from build123d import *

# Parameters (mm, degrees)
BOSS_EXTRUDE1_START                       = 12.7
BOSS_EXTRUDE1_DEPTH                       = 12.7
BOSS_EXTRUDE2_DEPTH                       = 12.7
SKETCH7_R                                 = 0.9525
CUT_EXTRUDE1_DEPTH                        = 111.090903984
SKETCH10_R                                = 0.9525
CUT_EXTRUDE2_DEPTH                        = 110.494104933
CSK_FOR_6_FLAT_HEAD_MACHINE_SCREW_2_COUNT = 2
CSK_FOR_6_FLAT_HEAD_MACHINE_SCREW_2_PITCH = 11.43


with BuildPart() as part:
    # Sweep1: sweep along a path in Sketch4
    with BuildLine(Plane.XY) as sweep1_path:
        Line((0, 0), (0, -92.964))
    # Sketch3 → Sweep1 (sweep)
    with BuildSketch(Plane(origin=(0, 0, 0), x_dir=(1, 0, 0), z_dir=(0, 1, 0))):
        with BuildLine():
            Line((0, 16.62500014), (-25.4, 16.62500014))
            Line((-25.4, 16.62500014), (-25.4, 10.27500014))
            Line((-25.4, 10.27500014), (-6.985, 10.27500014))
            ThreePointArc((-6.985, 10.27500014), (-6.535987194, 10.089012946), (-6.35, 9.64000014))
            Line((-6.35, 9.64000014), (-6.35, -14.48999986))
            ThreePointArc((-6.35, -14.48999986), (-6.535987194, -14.939012666), (-6.985, -15.12499986))
            Line((-6.985, -15.12499986), (-25.4, -15.12499986))
            Line((-25.4, -15.12499986), (-25.4, -21.47499986))
            Line((-25.4, -21.47499986), (0, -21.47499986))
            Line((0, -21.47499986), (0, 16.62500014))
        make_face()
    sweep(path=sweep1_path.line)

    # Sketch5 → Boss-Extrude1 (add)
    with BuildSketch(Plane.XZ.offset(92.964).offset(BOSS_EXTRUDE1_START)):
        with BuildLine():
            Line((-25.4, 18.04599986), (-3.429, 18.04599986))
            Line((-3.429, 18.04599986), (-3.429, -13.19600014))
            Line((-3.429, -13.19600014), (-25.4, -13.19600014))
            Line((-25.4, -13.19600014), (-25.4, -10.27500014))
            Line((-25.4, -10.27500014), (-6.985, -10.27500014))
            ThreePointArc((-6.985, -10.27500014), (-6.535987194, -10.089012946), (-6.35, -9.64000014))
            Line((-6.35, -9.64000014), (-6.35, 14.48999986))
            ThreePointArc((-6.35, 14.48999986), (-6.535987194, 14.939012666), (-6.985, 15.12499986))
            Line((-6.985, 15.12499986), (-25.4, 15.12499986))
            Line((-25.4, 15.12499986), (-25.4, 18.04599986))
        make_face()
    extrude(amount=-BOSS_EXTRUDE1_DEPTH)

    # Sketch6 → Boss-Extrude2 (add)
    with BuildSketch(Plane(origin=(0, 0, 0), x_dir=(1, 0, 0), z_dir=(0, 1, 0))):
        Polygon((-25.4, 13.45000014), (-25.4, 16.62500014), (0, 16.62500014), (0, -21.47499986), (-25.4, -21.47499986), (-25.4, -18.29999986), (-3.175, -18.29999986), (-3.175, 13.45000014), align=None)
    extrude(amount=BOSS_EXTRUDE2_DEPTH)

    # Sketch7 → Cut-Extrude1 (cut, through all)
    with BuildSketch(Plane.ZY.offset(3.175)):
        with Locations((-3.29000014, 6.35)):
            Circle(SKETCH7_R)
        with Locations((8.13999986, 6.35)):
            Circle(SKETCH7_R)
    extrude(amount=-CUT_EXTRUDE1_DEPTH, mode=Mode.SUBTRACT)

    # Sketch10 → Cut-Extrude2 (cut, through all)
    with BuildSketch(Plane.ZY.offset(6.35)):
        with Locations((-3.29000014, -99.314)):
            Circle(SKETCH10_R)
        with Locations((8.13999986, -99.314)):
            Circle(SKETCH10_R)
    extrude(amount=-CUT_EXTRUDE2_DEPTH, mode=Mode.SUBTRACT)

    # Sketch13 → CSK for #6 Flat Head Machine Screw (100)2 (revolve, cut)
    with BuildSketch(Plane(origin=(-6.35, -99.314, -3.29000014), x_dir=(0, 0, 1), z_dir=(0, 1, 0))):
        Polygon((0, 0), (0, 2.563442612), (2.15265, 1.27), (2.15265, 1.166893902), (3.5433, 0), align=None)
    csk_for_6_flat_head_machine_screw_100 = revolve(axis=Axis((-12.7, -99.314, -3.29000014), (1, 0, 0)), mode=Mode.SUBTRACT)

    # CSK for _6 Flat Head Machine Screw _ 2: CSK for #6 Flat Head Machine Screw (100)2 ×2
    with Locations(*[(0, 0, i * CSK_FOR_6_FLAT_HEAD_MACHINE_SCREW_2_PITCH) for i in range(1, CSK_FOR_6_FLAT_HEAD_MACHINE_SCREW_2_COUNT)]):
        add(csk_for_6_flat_head_machine_screw_100, mode=Mode.SUBTRACT)


solid = part.part
Model file for the job. Use its own axes, mm. A direction names the side the tool comes from. Coordinates: 2 decimals unless noted, no trailing zeros. Order: outer loops, then holes, each group sorted by start corner. A loop starts at its lowest first (then second) coordinate and runs counter-clockwise, first axis right, second up. Notation, with made-up numbers: M 64.5,3.25 L 79.5,3.25 A32 ccw 79.5,29.25 Z; hole C 43,2 d11. An arc over 180 degrees is marked long. Return JSON: item names as keys, results as strings.
1. Tool access for faces 1 (the face through (-3.175, 6, 3)), 2 (the face through (-3.429, -99, 3)), 3 (the face through (-6.35, -54, 2)): list every direction of +Z, -Z, +X, -X, +Y, -Y with a clear straight run to the whole face (end or side of a thin tool).
Ans:
{"face 1": "-X, +Y", "face 2": "+Z, -Z, +X, -Y", "face 3": "-X, +Y, -Y"}
2. Saw through at A-A (x = -9.25). Give the cut face in (y, z) (3 decimals).
Ans:
{"outline": "M -105.664,-13.196 L -92.964,-13.196 L -92.964,-16.625 L 12.7,-16.625 L 12.7,-13.45 L 0,-13.45 L 0,-10.275 L -105.664,-10.275 Z; M -105.664,15.125 L 0,15.125 L 0,18.3 L 12.7,18.3 L 12.7,21.475 L -92.964,21.475 L -92.964,18.046 L -105.664,18.046 Z"}
3. Pull direction Z, two halves, no side cores. Call faces 4 (the face through (-25.4, -47, 18)), 5 (the face through (-1.61, 5.99, 9.02)), 6 (the face through (-15, -99, 18.046)), 7 (the face through (-14, 6, 18.3)): +Z half, -Z half, draft (parallel to the pull), parting line (faces both ways), or undercut.
Ans:
{"face 4": "draft", "face 5": "undercut", "face 6": "+Z half", "face 7": "undercut"}
4. Flat gauge pins, fed straight in: pin 1 (3 mm diameter, centred on y = 6.35, z = -3.29, fed in from -X) (3 decimals); pin 2 (5 mm diameter, centred on y = -99.314, z = -3.29, fed in from +X); pin 3 (10 mm diameter, centred on x = -22.5, z = -8, fed in from +Y). Where does each tip first touch, or does it go through?
Ans:
{"pin 1": "x = -3.175", "pin 2": "x = -3.43", "pin 3": "y = 0"}
5. Drill centre lines: probe 1 along Y at (x, z) = (-0.85, -3.29); probe 2 along Z at (x, y) = (-19.25, -17) (3 decimals); probe 3 along Y at (x, z) = (-5.15, -3.29). Where is each one in solid material? Low to high.
Ans:
{"probe 1": "-92.96 to 5.4, 7.3 to 12.7", "probe 2": "-16.625 to -10.275, 15.125 to 21.475", "probe 3": "-105.66 to -101.47, -97.16 to 0"}
6. Saw through at B-B (z = 13). Give the cut face in (x, y) (3 decimals), and give its area (3 significant figures).
Ans:
{"outline": "M -6.35,-105.664 L -3.429,-105.664 L -3.429,-92.964 L 0,-92.964 L 0,12.7 L -3.175,12.7 L -3.175,0 L -6.35,0 Z", "area": "668 mm^2"}
7. Saw through at C-C (y = -69.5). Give the cut face in (x, z) (3 decimals).
Ans:
{"outline": "M -25.4,-16.625 L 0,-16.625 L 0,21.475 L -25.4,21.475 L -25.4,15.125 L -6.985,15.125 A0.635 cw -6.35,14.49 L -6.35,-9.64 A0.635 cw -6.985,-10.275 L -25.4,-10.275 Z"}
